Part model, mm, in its own coordinate system. A direction names the side the tool comes from. Give positions to 0.01 mm unless a question says otherwise; leave off trailing zeros. Order: outer loops, then holes, each group sorted by start corner. A loop starts at its lowest first (then second) coordinate and runs counter-clockwise, first axis right, second up.
1. Drop flat-ended pins along their axis: pin 1 Ø4.5 at (x, y) = (25.98, 15) entering from +Z; pin 2 Ø4.5 at (y, z) = (31.5, 26) entering from -X; pin 3 Ø8 at (x, z) = (43.5, 5) entering from +Y; pin 4 Ø2.5 at (y, z) = (-31.5, 26) entering from +X. Give the stop position or say it passes through.
2. Slice it at B-B on z = 9.5. List the corners of the cut face in (x, y).
3. Mould opens along Y. For faces 1 (the cylindrical face through (46.8, 33, 26.8)), 2 (the cylindrical face through (0.384, -32.925, 16.521)), 3 (the flat face through (-30, -38, 24)), 4 (the flat face through (26, -44.5, 24)) say: +Y half, -Y half, draft (parallel to the pull), parting line (faces both ways), or undercut.
4. Slice it at A-A on z = 37. List the corners of the cut face in (x, y).
5. Which spindle directions (+Z, -Z, +X, -X, +Y, -Y) get a long thin tool onto all of the face, cutting with end or side? Do faces 5 (the flat face through (-55, -32, 24)), 6 (the flat face through (45, 32, 24)), 7 (the cylindrical face through (-28, -21, 3)), 8 (the flat face through (-48.5, 31, 29)), 9 (the flat face through (-50, -20, 25)). Say none if no direction does.
6. Probe line 1 (Y direction, x = 54.35, z = 26); line 2 (Y direction, x = 0, z = 16.5); line 3 (Z direction, x = -53.8, y = 31.5). List the from-to ranges inside material, lowest first.
from build123d import *

# Parameters (mm, degrees)
SKETCH001_W                   = 10
SKETCH001_H                   = 23
PAD_DEPTH                     = 15
SKETCH002_R                   = 1.7
POCKET_DEPTH                  = 559.367976
POCKET001_DEPTH               = 1.5
SKETCH001_MIRRORED_2_W        = 10
SKETCH001_MIRRORED_2_H        = 23
PAD_MIRRORED_2_DEPTH          = 15
SKETCH002_MIRRORED_2_R        = 1.7
POCKET_MIRRORED_2_DEPTH       = 559.367976
POCKET001_MIRRORED_2_DEPTH    = 1.5
SKETCH004_R                   = 1.7
POCKET002_DEPTH               = 447.367976
SKETCH005_R                   = 2.95
POCKET003_DEPTH               = 3
POLARPATTERN_COUNT            = 3
PAD001_DEPTH                  = 25
POCKET004_DEPTH               = 13
SKETCH008_R                   = 1.7
POCKET005_DEPTH               = 10
POCKET006_DEPTH               = 5
PAD001_MIRRORED002_2_DEPTH    = 25
POCKET004_MIRRORED002_2_DEPTH = 13
SKETCH008_MIRRORED002_2_R     = 1.7
POCKET005_MIRRORED002_2_DEPTH = 10
POCKET006_MIRRORED002_2_DEPTH = 5


with BuildPart() as part:
    # Sketch → Revolution (revolve)
    with BuildSketch(Plane.XZ):
        Polygon((25, 0), (25, 18), (75, 18), (75, 13), (47, 13), (47, 6), (35, 6), (35, 0), align=None)
    revolve(axis=Axis((0, 0, 0), (0, 0, 1)))

    # Sketch001 (on Face2 of Revolution) → Pad (new body)
    with BuildSketch(Plane(origin=(0, 0, 18), x_dir=(-1, 0, 0), z_dir=(0, 0, 1))):
        with Locations((-50, -31.5)):
            Rectangle(SKETCH001_W, SKETCH001_H)
    pad = extrude(amount=PAD_DEPTH)

    # Sketch002 (on Face8 of Pad) → Pocket (cut, through all)
    with BuildSketch(Plane(origin=(55, 0, 0), x_dir=(0, 0, 1), z_dir=(1, 0, 0))):
        with Locations((26, -31.5)):
            Circle(SKETCH002_R)
    pocket = extrude(amount=-POCKET_DEPTH, mode=Mode.SUBTRACT)

    # Sketch003 (on DatumPlane) → Pocket001 (cut, symmetric)
    with BuildSketch(Plane(origin=(50, 0, 0), x_dir=(0, 0, 1), z_dir=(1, 0, 0))):
        Polygon((24.325, -28.598815), (22.65, -31.5), (24.325, -34.401185), (34.325, -34.401185), (34.325, -28.598815), align=None)
    pocket001 = extrude(amount=POCKET001_DEPTH, both=True, mode=Mode.SUBTRACT)

    # Sketch001 Mirrored 2 → Pad Mirrored 2 (add)
    with BuildSketch(Plane(origin=(0, 0, 18), x_dir=(-1, 0, 0), z_dir=(0, 0, -1))):
        with Locations((-50, -31.5)):
            Rectangle(SKETCH001_MIRRORED_2_W, SKETCH001_MIRRORED_2_H)
    pad_mirrored_2 = extrude(amount=-PAD_MIRRORED_2_DEPTH)

    # Sketch002 Mirrored 2 → Pocket Mirrored 2 (cut, through all)
    with BuildSketch(Plane.ZY.offset(-55)):
        with Locations((26, -31.5)):
            Circle(SKETCH002_MIRRORED_2_R)
    pocket_mirrored_2 = extrude(amount=POCKET_MIRRORED_2_DEPTH, mode=Mode.SUBTRACT)

    # Sketch003 Mirrored 2 → Pocket001 Mirrored 2 (cut, symmetric)
    with BuildSketch(Plane.ZY.offset(-50)):
        Polygon((24.325, -28.598815), (22.65, -31.5), (24.325, -34.401185), (34.325, -34.401185), (34.325, -28.598815), align=None)
    pocket001_mirrored_2 = extrude(amount=-POCKET001_MIRRORED_2_DEPTH, both=True, mode=Mode.SUBTRACT)

    # Mirrored001: Pad, Pocket, Pocket001, Pad Mirrored 2, Pocket Mirrored 2, Pocket001 Mirrored 2 across YZ
    add(pad.mirror(Plane.YZ))
    add(pocket.mirror(Plane.YZ), mode=Mode.SUBTRACT)
    add(pocket001.mirror(Plane.YZ), mode=Mode.SUBTRACT)
    add(pad_mirrored_2.mirror(Plane.YZ))
    add(pocket_mirrored_2.mirror(Plane.YZ), mode=Mode.SUBTRACT)
    add(pocket001_mirrored_2.mirror(Plane.YZ), mode=Mode.SUBTRACT)

    # Sketch004 (on Face3 of MultiTransform) → Pocket002 (cut, through all)
    with BuildSketch(Plane(origin=(0, 0, 18), x_dir=(-1, 0, 0), z_dir=(0, 0, 1))):
        with Locations((0, 30)):
            Circle(SKETCH004_R)
    pocket002 = extrude(amount=-POCKET002_DEPTH, mode=Mode.SUBTRACT)

    # Sketch005 (on Face3 of Pocket002) → Pocket003 (cut)
    with BuildSketch(Plane(origin=(0, 0, 18), x_dir=(-1, 0, 0), z_dir=(0, 0, 1))):
        with Locations((0, 30)):
            Circle(SKETCH005_R)
    pocket003 = extrude(amount=-POCKET003_DEPTH, mode=Mode.SUBTRACT)

    # PolarPattern: Pocket003, Pocket002 ×3 about axis
    polarpattern_axis = Axis((0, 0, 18), (0, 0, 1))
    for i in range(1, POLARPATTERN_COUNT):
        add(pocket003.rotate(polarpattern_axis, i * 360 / POLARPATTERN_COUNT), mode=Mode.SUBTRACT)
        add(pocket002.rotate(polarpattern_axis, i * 360 / POLARPATTERN_COUNT), mode=Mode.SUBTRACT)

    # Sketch006 (on Face3 of PolarPattern) → Pad001 (join)
    with BuildSketch(Plane(origin=(0, 0, 18), x_dir=(-1, 0, 0), z_dir=(0, 0, 1))):
        with BuildLine():
            Line((22, 66.452991), (22, 44.5))
            Line((22, 44.5), (30, 44.5))
            Line((30, 44.5), (30, 28))
            Line((30, 28), (17, 28))
            Line((17, 28), (17, 67.904344))
            ThreePointArc((22, 66.452991), (19.513498, 67.225169), (17, 67.904344))
        make_face()
    pad001 = extrude(amount=PAD001_DEPTH)

    # Sketch007 (on Face29 of Pad001) → Pocket004 (cut)
    with BuildSketch(Plane(origin=(-17, 0, 0), x_dir=(0, 0, 1), z_dir=(1, 0, 0))):
        Polygon((18, 28), (63, 73), (63, 28), align=None)
    pocket004 = extrude(amount=-POCKET004_DEPTH, mode=Mode.SUBTRACT)

    # Sketch008 (on Face30 of Pocket004) → Pocket005 (cut)
    with BuildSketch(Plane(origin=(0, -5, -5), x_dir=(1, 0, 0), z_dir=(0, 0.707107, 0.707107))):
        with Locations((-26, -50.726912)):
            Circle(SKETCH008_R)
    pocket005 = extrude(amount=-POCKET005_DEPTH, mode=Mode.SUBTRACT)

    # Sketch009 (on DatumPlane) → Pocket006 (cut)
    with BuildSketch(Plane(origin=(0, -6.414214, -6.414214), x_dir=(1, 0, 0), z_dir=(0, 0.707107, 0.707107))):
        Polygon((-24.325, -53.628097), (-22.65, -50.726912), (-24.325, -47.825727), (-27.675, -47.825727), (-29.35, -50.726912), (-27.675, -53.628097), align=None)
    pocket006 = extrude(amount=-POCKET006_DEPTH, mode=Mode.SUBTRACT)

    # Sketch006 Mirrored002 2 → Pad001 Mirrored002 2 (add)
    with BuildSketch(Plane(origin=(0, 0, 18), x_dir=(1, 0, 0), z_dir=(0, 0, -1))):
        with BuildLine():
            Line((22, 66.452991), (22, 44.5))
            Line((22, 44.5), (30, 44.5))
            Line((30, 44.5), (30, 28))
            Line((30, 28), (17, 28))
            Line((17, 28), (17, 67.904344))
            ThreePointArc((22, 66.452991), (19.513498, 67.225169), (17, 67.904344))
        make_face()
    pad001_mirrored002_2 = extrude(amount=-PAD001_MIRRORED002_2_DEPTH)

    # Sketch007 Mirrored002 2 → Pocket004 Mirrored002 2 (cut)
    with BuildSketch(Plane(origin=(17, 0, 0), x_dir=(0, 0, 1), z_dir=(1, 0, 0))):
        Polygon((18, 28), (63, 73), (63, 28), align=None)
    pocket004_mirrored002_2 = extrude(amount=POCKET004_MIRRORED002_2_DEPTH, mode=Mode.SUBTRACT)

    # Sketch008 Mirrored002 2 → Pocket005 Mirrored002 2 (cut)
    with BuildSketch(Plane(origin=(0, -5, -5), x_dir=(-1, 0, 0), z_dir=(0, -0.707107, -0.707107))):
        with Locations((-26, -50.726912)):
            Circle(SKETCH008_MIRRORED002_2_R)
    pocket005_mirrored002_2 = extrude(amount=POCKET005_MIRRORED002_2_DEPTH, mode=Mode.SUBTRACT)

    # Sketch009 Mirrored002 2 → Pocket006 Mirrored002 2 (cut)
    with BuildSketch(Plane(origin=(0, -6.414214, -6.414214), x_dir=(-1, 0, 0), z_dir=(0, -0.707107, -0.707107))):
        Polygon((-24.325, -53.628097), (-22.65, -50.726912), (-24.325, -47.825727), (-27.675, -47.825727), (-29.35, -50.726912), (-27.675, -53.628097), align=None)
    pocket006_mirrored002_2 = extrude(amount=POCKET006_MIRRORED002_2_DEPTH, mode=Mode.SUBTRACT)

    # Mirrored003: Pad001, Pocket004, Pocket005, Pocket006, Pad001 Mirrored002 2, Pocket004 Mirrored002 2, Pocket005 Mirrored002 2, Pocket006 Mirrored002 2 across Sketch006 H_Axis
    add(pad001.mirror(Plane(origin=(0, 0, 18), x_dir=(0, 0, 1), z_dir=(0, -1, 0))))
    add(pocket004.mirror(Plane(origin=(0, 0, 18), x_dir=(0, 0, 1), z_dir=(0, -1, 0))), mode=Mode.SUBTRACT)
    add(pocket005.mirror(Plane(origin=(0, 0, 18), x_dir=(0, 0, 1), z_dir=(0, -1, 0))), mode=Mode.SUBTRACT)
    add(pocket006.mirror(Plane(origin=(0, 0, 18), x_dir=(0, 0, 1), z_dir=(0, -1, 0))), mode=Mode.SUBTRACT)
    add(pad001_mirrored002_2.mirror(Plane(origin=(0, 0, 18), x_dir=(0, 0, 1), z_dir=(0, -1, 0))))
    add(pocket004_mirrored002_2.mirror(Plane(origin=(0, 0, 18), x_dir=(0, 0, 1), z_dir=(0, -1, 0))), mode=Mode.SUBTRACT)
    add(pocket005_mirrored002_2.mirror(Plane(origin=(0, 0, 18), x_dir=(0, 0, 1), z_dir=(0, -1, 0))), mode=Mode.SUBTRACT)
    add(pocket006_mirrored002_2.mirror(Plane(origin=(0, 0, 18), x_dir=(0, 0, 1), z_dir=(0, -1, 0))), mode=Mode.SUBTRACT)


solid = part.part
Data:
1. pin 1: stops at z = 15
1. pin 2: stops at x = -55
1. pin 3: stops at y = 25.27
1. pin 4: passes through
2. outline: circle Ø94 at (0, 0); hole circle Ø3.4 at (-25.98, 15); hole circle Ø50 at (0, 0); hole circle Ø3.4 at (0, -30); hole circle Ø3.4 at (25.98, 15)
3. face 1: undercut
3. face 2: undercut
3. face 3: draft
3. face 4: -Y half
4. outline: (-22, -66.45) arc R70 ccw to (-17, -67.9) - (-17, -47) - (-22, -47) - close; (-22, 47) - (-17, 47) - (-17, 67.9) arc R70 ccw to (-22, 66.45) - close; (17, -67.9) arc R70 ccw to (22, -66.45) - (22, -47) - (17, -47) - close; (17, 47) - (22, 47) - (22, 66.45) arc R70 ccw to (17, 67.9) - close
5. face 5: +Z, -X, +Y, -Y
5. face 6: +Z, +Y, -Y
5. face 7: -Z
5. face 8: +Z
5. face 9: +Z, +X, -X
6. line 1: y = -43 to -33.2, -29.8 to -20, 20 to 29.8, 33.2 to 43
6. line 2: y = -75 to -32.95, -27.05 to -25, 25 to 75
6. line 3: z = 13 to 24.3, 27.7 to 33
